from build123d import *

# Parameters (mm, degrees)
ESQUISSE1_W             = 35.68
ESQUISSE1_H             = 21.82
BOSS_EXTRU_1_DEPTH      = 6
ESQUISSE2_W             = 33.68
ESQUISSE2_H             = 19.82
ENL_V_MAT_EXTRU_1_DEPTH = 5
ESQUISSE3_W             = 32.68
ESQUISSE3_H             = 18.82
ENL_V_MAT_EXTRU_2_DEPTH = 43.120954405
ESQUISSE4_W             = 4
ESQUISSE4_H             = 16.82
ENL_V_MAT_EXTRU_3_DEPTH = 5


with BuildPart() as part:
    # Esquisse1 → Boss.-Extru.1 (new body)
    with BuildSketch(Plane.XY):
        with Locations((17.84, 10.91)):
            Rectangle(ESQUISSE1_W, ESQUISSE1_H)
    extrude(amount=BOSS_EXTRU_1_DEPTH)

    # Esquisse2 → Enlèv. mat.-Extru.1 (cut)
    with BuildSketch(Plane.XY.offset(6)):
        with Locations((17.84, 10.91)):
            Rectangle(ESQUISSE2_W, ESQUISSE2_H)
    extrude(amount=-ENL_V_MAT_EXTRU_1_DEPTH, mode=Mode.SUBTRACT)

    # Esquisse3 → Enlèv. mat.-Extru.2 (cut, through all)
    with BuildSketch(Plane.XY.offset(1)):
        with Locations((17.84, 10.91)):
            Rectangle(ESQUISSE3_W, ESQUISSE3_H)
    extrude(amount=-ENL_V_MAT_EXTRU_2_DEPTH, mode=Mode.SUBTRACT)

    # Esquisse4 → Enlèv. mat.-Extru.3 (cut)
    with BuildSketch(Plane(origin=(35.68, 0, 0), x_dir=(0, 0, -1), z_dir=(1, 0, 0))):
        with Locations((-4, 10.41)):
            Rectangle(ESQUISSE4_W, ESQUISSE4_H)
    extrude(amount=-ENL_V_MAT_EXTRU_3_DEPTH, mode=Mode.SUBTRACT)


solid = part.part
The model under review builds one solid part; all positions refer to its coordinate system, in mm. A direction names the side the tool comes from. Give positions to 0.01 mm unless a question says otherwise; leave off trailing zeros. Write each loop counter-clockwise with the first axis right and the second up, starting at its lowest first coordinate (ties: lowest second). Pieces come first, ordered by that corner, then holes. Notation, with made-up numbers: M 44,-37 L 66,-37 A3 ccw 66,-32 Z; hole C -15.5,26 d7. An arc over 180 degrees is marked long. One line per question, with ' | ' between items. Start each with the question number.
Item 1: We need section B-B on z = 1.4. Write out the cut boundary in (x, y).
Item 2: For pin 1 (1.1 mm diameter, centred on x = 35.5, z = 3.5, fed in from -Y); pin 2 (8 mm diameter, centred on x = 21, y = 14.5, fed in from -Z); pin 3 (1.5 mm diameter, centred on y = 11.5, z = 3.5, fed in from +X), all flat-tipped, find the tip position at first contact; note any pin that passes through.
Item 3: Wall thickness on line 1 (Y direction, x = 4.5, z = 4.6); line 2 (X direction, y = 2, z = 1.5); line 3 (X direction, y = 17.75, z = 0.35): over which ranges is each line inside the solid? List them lowest first. Write a range as from..to.
Item 4: For faces 5 (the flat face through (17.6, 1.5, 0.5)), 6 (the flat face through (34.68, 10.8, 1.3)), 7 (the flat face through (35, 10, 2)), 8 (the flat face through (18, 0, 3)), list the 3-axis set-ups (+Z, -Z, +X, -X, +Y, -Y) from which the entire face can be reached by the end or side of a thin tool; tool diameter is ignored.
Item 5: Draft analysis for pull direction X (two halves, no side actions). For faces 1 (the flat face through (35, 2, 4)), 2 (the flat face through (34.18, 10.8, 0.5)), 3 (the flat face through (0, 11, 3)), 4 (the flat face through (18, 20.82, 4)), state which applies: released by +X, released by -X, zero draft, split by the parting line, or undercut.
Item 6: We need section C-C on x = 31. Write out the cut boundary in (y, z).
Item 7: We need section A-A on y = 3.25. Write out the cut boundary in (x, z), plus the area to 3 significant figures.
Results found:
1) outline: M 0,0 L 35.68,0 L 35.68,21.82 L 0,21.82 Z; hole M 1,1 L 34.68,1 L 34.68,20.82 L 1,20.82 Z
2) pin 1: stops at y = 0 | pin 2: passes through | pin 3: stops at x = 1
3) line 1: y = 0..1, 20.82..21.82 | line 2: x = 0..1, 34.68..35.68 | line 3: x = 0..1.5, 34.18..35.68
4) face 5: +Z, -Z | face 6: +Z | face 7: +Z, +X | face 8: +Z, -Z, +X, -X, -Y
5) face 1: zero draft | face 2: undercut | face 3: released by -X | face 4: undercut
6) outline: M 0,0 L 1.5,0 L 1.5,1 L 1,1 L 1,6 L 0,6 Z; M 20.32,0 L 21.82,0 L 21.82,6 L 20.82,6 L 20.82,1 L 20.32,1 Z
7) outline: M 0,0 L 1.5,0 L 1.5,1 L 1,1 L 1,6 L 0,6 Z; M 34.18,0 L 35.68,0 L 35.68,2 L 34.68,2 L 34.68,1 L 34.18,1 Z | area: 9.00 mm2
